Verification items for the finished model (mm, model axes). Give positions to 0.01 mm unless a question says otherwise; leave off trailing zeros. Write each loop counter-clockwise with the first axis right and the second up, starting at its lowest first coordinate (ties: lowest second). Pieces come first, ordered by that corner, then holes. Notation, with made-up numbers: (3, -7) -> (27, -7) arc R22 cw to (27, 32) -> close; hole circle Ø10 at (83.25, 55). An arc over 180 degrees is marked (long way). Answer as CSV lines item,"result". Start each with the question number.
1) Material ranges on L1, parallel to Y at x = 8.25, z = 0; L2, parallel to Y at x = 15, z = -19.5; L3, parallel to Z at x = 6, y = -81, recorded low to high.
2) Sectioned sample at A-A on y = -101.6. Record the cut outline in (x, z), and give its area (3 significant figures).
3) Mould release check, pull along Z, two halves, no side actions. Record for faces 1 (the flat face through (13, -152.4, 2)), 2 (the flat face through (13, 73, 152.4)), 3 (the cylindrical face through (12.522, -126.396, -5.506)): released by +Z, released by -Z, zero draft, split by the parting line, or undercut.
4) Sectioned sample at B-B on z = 0. Record the cut outline in (x, y).
```python
from build123d import *

# Parameters (mm, degrees)
SKETCH1_W           = 304.8
SKETCH1_H           = 304.8
BOSS_EXTRUDE1_DEPTH = 25.4
SKETCH2_R           = 25.4
CUT_EXTRUDE1_DEPTH  = 25.4
SKETCH3_W           = 25.4
SKETCH3_H           = 304.8
BOSS_EXTRUDE2_DEPTH = 152.4


with BuildPart() as part:
    # Sketch1 → Boss-Extrude1 (new body)
    with BuildSketch(Plane(origin=(0, 0, 0), x_dir=(0, 0, -1), z_dir=(1, 0, 0))):
        Rectangle(SKETCH1_W, SKETCH1_H)
    extrude(amount=BOSS_EXTRUDE1_DEPTH)

    # Sketch2 → Cut-Extrude1 (cut)
    with BuildSketch(Plane.ZY):
        with Locations((0, -101.6)):
            Circle(SKETCH2_R)
    extrude(amount=-CUT_EXTRUDE1_DEPTH, mode=Mode.SUBTRACT)

    # Sketch3 → Boss-Extrude2 (add)
    with BuildSketch(Plane(origin=(0, 152.4, 0), x_dir=(1, 0, 0), z_dir=(0, 1, 0))):
        with Locations((12.7, 0)):
            Rectangle(SKETCH3_W, SKETCH3_H)
    extrude(amount=BOSS_EXTRUDE2_DEPTH)


solid = part.part
```
Ans:
1,L1,"y = -152.4 to -127, -76.2 to 304.8"
1,L2,"y = -152.4 to -117.88, -85.32 to 304.8"
1,L3,"z = -152.4 to -14.86, 14.86 to 152.4"
2,outline,"(0, -152.4) -> (25.4, -152.4) -> (25.4, -25.4) -> (0, -25.4) -> close; (0, 25.4) -> (25.4, 25.4) -> (25.4, 152.4) -> (0, 152.4) -> close"
2,area,"6,450 mm²"
3,face 1,"zero draft"
3,face 2,"released by +Z"
3,face 3,"undercut"
4,outline,"(0, -152.4) -> (25.4, -152.4) -> (25.4, -127) -> (0, -127) -> close; (0, -76.2) -> (25.4, -76.2) -> (25.4, 304.8) -> (0, 304.8) -> close"
